```python
from build123d import *

# Parameters (mm, degrees)
MAINBASESKETCH_W             = 15.8
MAINBASESKETCH_H             = 3.2
MAINBASEEXTRUDE_DEPTH        = 7.9
LCUTBLUE_DEPTH               = 19.555463972
LCUTBLUE_DEPTH_BACK          = 19.555463972
MADESLIMCUTSKETCH_W          = 7.9
MADESLIMCUTSKETCH_H          = 7.9
MADESLIMCUT_DEPTH            = 19.555463972
SHORTLEXTENSIONSKETCH_W      = 1.583745828
SHORTLEXTENSIONSKETCH_H      = 7.9
SHORTLUPPERCIRCLES_START     = -0.2
SHORTLUPPERCIRCLESSKETCH_R   = 2.45
SHORTLUPPERCIRCLESSKETCH_R_2 = 2
SHORTLUPPERCIRCLES_DEPTH     = 2
SHELL1_START                 = 1.2
SHELL1_OUTLINE_W             = 13.4
SHELL1_OUTLINE_H             = 7.083745828
SHELL1_DEPTH                 = 2
BOSS_EXTRUDE4_REACH          = 21.272
BOSS_EXTRUDE4_START          = -0.4
SKETCH89_R                   = 1.5
SKETCH89_R_2                 = 0.75
SKETCH89_W                   = 0.996828099
SKETCH89_H                   = 1
SKETCH89_W_2                 = 0.996828098
SKETCH90_R                   = 2.4
BOSS_EXTRUDE5_DEPTH          = 1.5


# Read off the part's stored shape, not the designer's step: Shell1
with BuildPart() as part:
    # MainBaseSketch → MainBaseExtrude (new, symmetric)
    with BuildSketch(Plane.XY):
        with Locations((8.581967213, 1.6)):
            Rectangle(MAINBASESKETCH_W, MAINBASESKETCH_H)
    extrude(amount=MAINBASEEXTRUDE_DEPTH, both=True)

    # LCUTBlueSketch → LCutBlue (cut, two sides: drawn at the far end of the back side and taken through both)
    with BuildSketch(Plane(origin=(0, 3.2, 0), x_dir=(1, 0, 0), z_dir=(0, 1, 0)).offset(-LCUTBLUE_DEPTH_BACK)):
        Polygon((8.581967213, 53.229874044), (8.581967213, 7.9), (8.581967213, 0), (16.481967213, 0), (61.811841258, 0), (125.917963912, 64.106122654), (72.688089868, 117.335996699), align=None)
    extrude(amount=LCUTBLUE_DEPTH + LCUTBLUE_DEPTH_BACK, mode=Mode.SUBTRACT)

    # MadeSlimCutSketch → MadeSlimCut (cut, through all)
    with BuildSketch(Plane.XZ):
        with Locations((4.631967213, -3.95)):
            Rectangle(MADESLIMCUTSKETCH_W, MADESLIMCUTSKETCH_H)
    extrude(amount=-MADESLIMCUT_DEPTH, mode=Mode.SUBTRACT)

    # ShortLExtension: sweep along a curve in space
    with BuildLine() as shortlextension_path:
        Line((0.681967213, 3.2, 0), (16.481967213, 3.2, 0))
    # ShortLExtensionSketch → ShortLExtension (sweep)
    with BuildSketch(Plane(origin=(16.481967213, 0, 0), x_dir=(0, 0, -1), z_dir=(1, 0, 0))):
        with Locations((0.791872914, 3.95)):
            Rectangle(SHORTLEXTENSIONSKETCH_W, SHORTLEXTENSIONSKETCH_H)
    sweep(path=shortlextension_path.line)

    # ShortLUpperCirclesSketch → ShortLUpperCircles (add)
    # profile 1 of 2: a face of its own
    with BuildSketch(Plane(origin=(0, 0, -1.583745828), x_dir=(-1, 0, 0), z_dir=(0, 0, -1)).offset(SHORTLUPPERCIRCLES_START)):
        with Locations(Location((-12.581967213, 3.95, 0), (0, 0, 90))):
            Circle(SHORTLUPPERCIRCLESSKETCH_R)
        with Locations(Location((-12.581967213, 3.95, 0), (0, 0, 90))):
            Circle(SHORTLUPPERCIRCLESSKETCH_R_2, mode=Mode.SUBTRACT)
    # profile 2 of 2: a face of its own
    with BuildSketch(Plane(origin=(0, 0, -1.583745828), x_dir=(-1, 0, 0), z_dir=(0, 0, -1)).offset(SHORTLUPPERCIRCLES_START)):
        with Locations(Location((-4.581967213, 3.95, 0), (0, 0, 270))):
            Circle(SHORTLUPPERCIRCLESSKETCH_R)
        with Locations(Location((-4.581967213, 3.95, 0), (0, 0, 270))):
            Circle(SHORTLUPPERCIRCLESSKETCH_R_2, mode=Mode.SUBTRACT)
    extrude(amount=SHORTLUPPERCIRCLES_DEPTH)

    # Shell1 outline → Shell1 (cut)
    with BuildSketch(Plane(origin=(0, 0, 0), x_dir=(1, 0, 0), z_dir=(0, 1, 0)).offset(SHELL1_START)):
        with Locations((8.581967213, -3.158127086)):
            Rectangle(SHELL1_OUTLINE_W, SHELL1_OUTLINE_H)
    extrude(amount=SHELL1_DEPTH, mode=Mode.SUBTRACT)

    # Sketch89 → Boss-Extrude4 (add, up to next)
    with BuildSketch(Plane(origin=(0, 3.2, 0), x_dir=(1, 0, 0), z_dir=(0, 1, 0)).offset(BOSS_EXTRUDE4_START), mode=Mode.PRIVATE) as boss_extrude4_sk1:
        with Locations(Location((8.581967213, -3.158127086, 0), (0, 0, 270))):
            Circle(SKETCH89_R)
        with Locations(Location((8.581967213, -3.158127086, 0), (0, 0, 270))):
            Circle(SKETCH89_R_2, mode=Mode.SUBTRACT)
    boss_extrude4_tool1 = extrude(boss_extrude4_sk1.sketch, amount=-BOSS_EXTRUDE4_REACH, mode=Mode.PRIVATE) - part.part
    # Sketch89 → Boss-Extrude4 (add, up to next)
    with BuildSketch(Plane(origin=(0, 3.2, 0), x_dir=(1, 0, 0), z_dir=(0, 1, 0)).offset(BOSS_EXTRUDE4_START), mode=Mode.PRIVATE) as boss_extrude4_sk2:
        with Locations((4.498879862, -0.5)):
            Rectangle(SKETCH89_W, SKETCH89_H)
    boss_extrude4_tool2 = extrude(boss_extrude4_sk2.sketch, amount=-BOSS_EXTRUDE4_REACH, mode=Mode.PRIVATE) - part.part
    # Sketch89 → Boss-Extrude4 (add, up to next)
    with BuildSketch(Plane(origin=(0, 3.2, 0), x_dir=(1, 0, 0), z_dir=(0, 1, 0)).offset(BOSS_EXTRUDE4_START), mode=Mode.PRIVATE) as boss_extrude4_sk3:
        with Locations((8.609734638, -0.5)):
            Rectangle(SKETCH89_W_2, SKETCH89_H)
    boss_extrude4_tool3 = extrude(boss_extrude4_sk3.sketch, amount=-BOSS_EXTRUDE4_REACH, mode=Mode.PRIVATE) - part.part
    # Sketch89 → Boss-Extrude4 (add, up to next)
    with BuildSketch(Plane(origin=(0, 3.2, 0), x_dir=(1, 0, 0), z_dir=(0, 1, 0)).offset(BOSS_EXTRUDE4_START), mode=Mode.PRIVATE) as boss_extrude4_sk4:
        with Locations((12.499284685, -0.5)):
            Rectangle(SKETCH89_W_2, SKETCH89_H)
    boss_extrude4_tool4 = extrude(boss_extrude4_sk4.sketch, amount=-BOSS_EXTRUDE4_REACH, mode=Mode.PRIVATE) - part.part
    add(boss_extrude4_tool1.solids().sort_by_distance((8.581967, 2.8, 1.700553))[0])
    add(boss_extrude4_tool2.solids().sort_by_distance((4.49888, 2.8, 0.5))[0])
    add(boss_extrude4_tool3.solids().sort_by_distance((8.609735, 2.8, 0.5))[0])
    add(boss_extrude4_tool4.solids().sort_by_distance((12.499285, 2.8, 0.5))[0])

    # Sketch90 → Boss-Extrude5 (add)
    with BuildSketch(Plane(origin=(0, 0, 0), x_dir=(-1, 0, 0), z_dir=(0, -1, 0))):
        with Locations(Location((-12.581967213, -3.158127086, 0), (0, 0, 270))):
            Circle(SKETCH90_R)
        with Locations(Location((-4.581967213, -3.158127086, 0), (0, 0, 270))):
            Circle(SKETCH90_R)
    extrude(amount=BOSS_EXTRUDE5_DEPTH)


solid = part.part
```
The model under review builds one solid part; all positions refer to its coordinate system, in mm. A direction names the side the tool comes from. Round coordinates to 2 decimals unless told otherwise and drop trailing zeros. Loops run counter-clockwise (first coordinate to the right, second up) from the corner with the lowest first, then second, coordinate; pieces in that order, holes last. Notation, with made-up numbers: (22.5, -25.5) - (55.5, -25.5) arc R32 ccw to (55.5, 7.5) - close; hole circle Ø6 at (75, -30.75). An arc over 180 degrees is marked (long way). Write each question's results on one line, items separated by ' | '. Start each with the question number.
Q1. Insertion check: P1, Ø4, axis at x = 9, z = 5.5, coming from the +Y side; P2, Ø1.4, axis at x = 8.5, y = 6, coming from the +Z side; P3, Ø1, axis at x = 14, z = 5.5, coming from the +Y side. Each pin has a flat end and moves straight along its axis. Give the tip position at first contact, or say it passes through.
Q2. Wall thickness on line 1 along X through (y, z) = (3.95, -2.5); line 2 along Y through (x, z) = (4.5, -2.5); line 3 along Z through (x, y) = (9.5, 2.5): over which ranges is each line inside the solid? List them lowest first. Write a range as [from, to].
Q3. Take a section at C-C on x = 3.25. Give the boundary of the cut face in (y, z).
Q4. Take a section at A-A on y = 3.95. Give the boundary of the cut face in (x, z).
Q5. Tool access review of faces 4 (the flat face through (12.5, 2, 0)), 5 (the cylindrical face through (10.07, 2.01, 2.96)), 6 (the flat face through (9, 4, -1.584)): name each direction out of +Z, -Z, +X, -X, +Y, -Y from which nothing blocks a thin tool from reaching the whole face with its end or side.
Q6. Draft analysis for pull direction X (two halves, no side actions). For faces 1 (the flat face through (8, 2.8, 2)), 2 (the flat face through (9, 6, 0)), 3 (the flat face through (0.682, 2, 2)), state which applies: pulls with the +X half, pulls with the -X half, needs draft (parallel to the pull), parting line crosses it, or undercut.
Q7. Take a section at B-B on z = 7.25. Give the boundary of the cut face in (x, y).
Q8. Take a section at D-D on y = 2.25. Give the number of separate pieces and of enclosed holes in the cut face, plus the area to 3 significant figures.
Data:
1) P1: stops at y = 3.2 | P2: stops at z = 0 | P3: stops at y = 1.2
2) line 1: x = [2.13, 2.58], [6.58, 7.03], [10.13, 10.58], [14.58, 15.03] | line 2: y = [1.5, 1.95], [5.95, 6.4] | line 3: z = [-1.58, -0.38], [1.97, 4.34], [6.7, 7.9]
3) outline: (-1.5, 1.16) - (0, 1.16) - (0, -1.58) - (1.89, -1.58) - (1.89, -3.38) - (2.46, -3.38) - (2.46, -1.58) - (5.44, -1.58) - (5.44, -3.38) - (6.01, -3.38) - (6.01, -1.58) - (7.9, -1.58) - (7.9, 0) - (3.2, 0) - (3.2, -0.38) - (1.2, -0.38) - (1.2, 6.7) - (3.2, 6.7) - (3.2, 7.9) - (0, 7.9) - (0, 5.15) - (-1.5, 5.15) - close
4) outline: (0.68, -1.58) - (2.13, -1.58) - (2.13, -3.38) - (2.58, -3.38) - (2.58, -1.58) - (6.58, -1.58) - (6.58, -3.38) - (7.03, -3.38) - (7.03, -1.58) - (10.13, -1.58) - (10.13, -3.38) - (10.58, -3.38) - (10.58, -1.58) - (14.58, -1.58) - (14.58, -3.38) - (15.03, -3.38) - (15.03, -1.58) - (16.48, -1.58) - (16.48, 0) - (0.68, 0) - close
5) face 4: none | face 5: +Y | face 6: -Z
6) face 1: undercut | face 2: needs draft | face 3: pulls with the -X half
7) outline: (0.68, 0) - (16.48, 0) - (16.48, 3.2) - (0.68, 3.2) - close
8) separate pieces: 5 | enclosed holes: 2 | area: 68.3 mm²
